Could you check a few things on this model? Use its own coordinates, in mm. A direction names the side the tool comes from. Give positions to 0.01 mm unless a question says otherwise; leave off trailing zeros. Write each loop counter-clockwise with the first axis right and the second up, starting at its lowest first coordinate (ties: lowest second). Pieces come first, ordered by that corner, then holes. Notation, with made-up numbers: (-28, 58.25) - (-4, 58.25) arc R15 ccw to (-4, 69.25) - close; hole circle Ø3 at (43.5, 58.5). An arc over 180 degrees is marked (long way). Use one line per item in the form item = value.
```python
from build123d import *

# Parameters (mm, degrees)
F0_W     = 54
F0_H     = 85
F1_DEPTH = 2
F2_DEPTH = 2
F3_W     = 26
F3_H     = 25
F3_W_2   = 25
F3_H_2   = 24
F4_DEPTH = 3
F3_W_3   = 8.1
F3_H_3   = 4.05
F5_DEPTH = 2
F6_R     = 0.5


with BuildPart() as f1:
    # F0 (on Top) → F1 (new body)
    with BuildSketch(Plane.XY):
        with BuildLine():
            Line((-30.5, 44), (-30.5, 0))
            Line((-30.5, 0), (-30.5, -44))
            ThreePointArc((-30.5, -44), (-29.9142135624, -45.4142135624), (-28.5, -46))
            Line((-28.5, -46), (28.5, -46))
            ThreePointArc((28.5, -46), (29.9142135624, -45.4142135624), (30.5, -44))
            Line((30.5, -44), (30.5, 0))
            Line((30.5, 0), (30.5, 44))
            ThreePointArc((30.5, 44), (29.9142135624, 45.4142135624), (28.5, 46))
            Line((28.5, 46), (-28.5, 46))
            ThreePointArc((-28.5, 46), (-29.9142135624, 45.4142135624), (-30.5, 44))
        make_face()
        with BuildLine():
            Line((-28.5, -42), (-28.5, 0))
            Line((-28.5, 0), (-28.5, 42))
            ThreePointArc((-28.5, 42), (-27.9142135624, 43.4142135624), (-26.5, 44))
            Line((-26.5, 44), (26.5, 44))
            ThreePointArc((26.5, 44), (27.9142135624, 43.4142135624), (28.5, 42))
            Line((28.5, 42), (28.5, 0))
            Line((28.5, 0), (28.5, -42))
            ThreePointArc((28.5, -42), (27.9142135624, -43.4142135624), (26.5, -44))
            Line((26.5, -44), (-26.5, -44))
            ThreePointArc((-26.5, -44), (-27.9142135624, -43.4142135624), (-28.5, -42))
        make_face(mode=Mode.SUBTRACT)
        with BuildLine():
            Line((-28.5, 42), (-28.5, 0))
            Line((-28.5, 0), (-28.5, -42))
            ThreePointArc((-28.5, -42), (-27.9142135624, -43.4142135624), (-26.5, -44))
            Line((-26.5, -44), (26.5, -44))
            ThreePointArc((26.5, -44), (27.9142135624, -43.4142135624), (28.5, -42))
            Line((28.5, -42), (28.5, 0))
            Line((28.5, 0), (28.5, 42))
            ThreePointArc((28.5, 42), (27.9142135624, 43.4142135624), (26.5, 44))
            Line((26.5, 44), (-26.5, 44))
            ThreePointArc((-26.5, 44), (-27.9142135624, 43.4142135624), (-28.5, 42))
        make_face()
        Rectangle(F0_W, F0_H, mode=Mode.SUBTRACT)
        Rectangle(F0_W, F0_H)
    extrude(amount=-F1_DEPTH)

    # F0 (on Top) → F2 (join)
    with BuildSketch(Plane.XY):
        with BuildLine():
            Line((-28.5, 42), (-28.5, 0))
            Line((-28.5, 0), (-28.5, -42))
            ThreePointArc((-28.5, -42), (-27.9142135624, -43.4142135624), (-26.5, -44))
            Line((-26.5, -44), (26.5, -44))
            ThreePointArc((26.5, -44), (27.9142135624, -43.4142135624), (28.5, -42))
            Line((28.5, -42), (28.5, 0))
            Line((28.5, 0), (28.5, 42))
            ThreePointArc((28.5, 42), (27.9142135624, 43.4142135624), (26.5, 44))
            Line((26.5, 44), (-26.5, 44))
            ThreePointArc((-26.5, 44), (-27.9142135624, 43.4142135624), (-28.5, 42))
        make_face()
        Rectangle(F0_W, F0_H, mode=Mode.SUBTRACT)
    extrude(amount=F2_DEPTH)

    # F3 (on Top) → F4 (join)
    with BuildSketch(Plane.XY):
        with Locations((0, 22.95)):
            Rectangle(F3_W, F3_H)
        with Locations((0, 22.95)):
            Rectangle(F3_W_2, F3_H_2, mode=Mode.SUBTRACT)
    extrude(amount=F4_DEPTH)

    # F3 (on Top) → F5 (cut, through all)
    with BuildSketch(Plane.XY):
        with Locations((0, 18.425)):
            Rectangle(F3_W_3, F3_H_3)
        with Locations((0, 22.475)):
            Rectangle(F3_W_3, F3_H_3)
    extrude(amount=-F5_DEPTH, mode=Mode.SUBTRACT)

    # F6
    f6_edges = [f1.edges().sort_by_distance(p)[0] for p in [
        (-12.5, 22.95, 0),
        (0, 10.95, 0),
        (0, 34.95, 0),
        (12.5, 22.95, 0),
        (0, 16.4, 0),
        (4.05, 20.45, 0),
        (0, 24.5, 0),
        (-4.05, 20.45, 0),
        (-27, 0, 0),
        (0, -42.5, 0),
        (0, 42.5, 0),
        (27, 0, 0),
        (0, 35.45, 0),
        (-13, 22.95, 0),
        (0, 10.45, 0),
        (13, 22.95, 0),
    ]]
    fillet(f6_edges, radius=F6_R)


solid = f1.part
```
1. If we mould it in two halves opening along Y, with no side actions, what happens to faces 6 (the face through (29.93, 45.4, -0.99)), 7 (the face through (0, 1, -2)), 8 (the face through (0, 35.45, 2)), 9 (the face through (27.9, -43.43, 0.99))? For each: pulls with the +Y half, pulls with the -Y half, needs draft (parallel to the pull), parting line crosses it, or undercut.
Response values:
face_6 = pulls with the +Y half
face_7 = needs draft
face_8 = undercut
face_9 = pulls with the -Y half
2. Imagine slicing it at D-D, the plane y = 26. List the corners of the cut face in (x, z) for me, and give its area (3 significant figures).
Response values:
outline = (-30.5, -2) - (30.5, -2) - (30.5, 0) - (28.5, 0) - (28.5, 2) - (27, 2) - (27, 0.5) arc R0.5 cw to (26.5, 0) - (13.5, 0) arc R0.5 cw to (13, 0.5) - (13, 3) - (12.5, 3) - (12.5, 0.5) arc R0.5 cw to (12, 0) - (-12, 0) arc R0.5 cw to (-12.5, 0.5) - (-12.5, 3) - (-13, 3) - (-13, 0.5) arc R0.5 cw to (-13.5, 0) - (-26.5, 0) arc R0.5 cw to (-27, 0.5) - (-27, 2) - (-28.5, 2) - (-28.5, 0) - (-30.5, 0) - close
area = 131 mm²
3. Which directions (+Z, -Z, +X, -X, +Y, -Y) give clear straight access to the entire face, cutting with the end or side of a thin tool? Please do faces 1 (the face through (28.5, -1, 1)), 2 (the face through (0, -44, 1)), 3 (the face through (-27.93, -43.4, 0.99)), 4 (the face through (-13, 23, 2)), 5 (the face through (0, 44, 1)).
Response values:
face_1 = +Z, +X, +Y, -Y
face_2 = +Z, +X, -X, -Y
face_3 = +Z, -X, -Y
face_4 = +Z
face_5 = +Z, +X, -X, +Y
4. Imagine slicing it at B-B, the plane x = -7. List the corners of the cut face in (y, z) for me, and give its area (3 significant figures).
Response values:
outline = (-46, -2) - (46, -2) - (46, 0) - (44, 0) - (44, 2) - (42.5, 2) - (42.5, 0.5) arc R0.5 cw to (42, 0) - (35.95, 0) arc R0.5 cw to (35.45, 0.5) - (35.45, 3) - (34.95, 3) - (34.95, 0.5) arc R0.5 cw to (34.45, 0) - (11.45, 0) arc R0.5 cw to (10.95, 0.5) - (10.95, 3) - (10.45, 3) - (10.45, 0.5) arc R0.5 cw to (9.95, 0) - (-42, 0) arc R0.5 cw to (-42.5, 0.5) - (-42.5, 2) - (-44, 2) - (-44, 0) - (-46, 0) - close
area = 193 mm²
5. For pin 1 (3 mm diameter, centred on x = -5.5, z = 2.5, fed in from -Y); pin 2 (1.6 mm diameter, centred on y = -8, z = 1, fed in from +X); pin 3 (1 mm diameter, centred on y = -31.5, z = 2, fed in from -X), each with a flat end and sliding along its axis, tell me the tip position at first contact or that it passes through.
Response values:
pin_1 = -44
pin_2 = 28.5
pin_3 = -28.5
6. Imagine slicing it at A-A, the plane y = -4.5. List the corners of the cut face in (x, z) for me, and give its area (3 significant figures).
Response values:
outline = (-30.5, -2) - (30.5, -2) - (30.5, 0) - (28.5, 0) - (28.5, 2) - (27, 2) - (27, 0.5) arc R0.5 cw to (26.5, 0) - (-26.5, 0) arc R0.5 cw to (-27, 0.5) - (-27, 2) - (-28.5, 2) - (-28.5, 0) - (-30.5, 0) - close
area = 128 mm²
7. Imagine slicing it at C-C, the plane x = 18. List the corners of the cut face in (y, z) for me, and give its area (3 significant figures).
Response values:
outline = (-46, -2) - (46, -2) - (46, 0) - (44, 0) - (44, 2) - (42.5, 2) - (42.5, 0.5) arc R0.5 cw to (42, 0) - (-42, 0) arc R0.5 cw to (-42.5, 0.5) - (-42.5, 2) - (-44, 2) - (-44, 0) - (-46, 0) - close
area = 190 mm²
8. If I drill on line 1 (Y direction, x = -6.5, z = 1.55); line 2 (X direction, y = 35, z = 0.7); line 3 (X direction, y = -1, z = 0.35), over which ranges is the centre line in solid material (lowest first)? Write a range as from..to.
Response values:
line_1 = -44..-42.5, 10.45..10.95, 34.95..35.45, 42.5..44
line_2 = -28.5..-27, -13..13, 27..28.5
line_3 = -28.5..-26.98, 26.98..28.5
